Design review of the part built by this model. Coordinates are the model's own, in mm. A direction names the side the tool comes from. Give positions to 0.01 mm unless a question says otherwise; leave off trailing zeros. Order: outer loops, then holes, each group sorted by start corner. A loop starts at its lowest first (then second) coordinate and runs counter-clockwise, first axis right, second up. Notation, with made-up numbers: M 31,15 L 90,15 A37 cw 90,52 Z; hole C 85.5,-25.75 d9. An arc over 180 degrees is marked long. Answer as a JSON object with one key per item and string values.
from build123d import *

# Parameters (mm, degrees)
CREATE_PROFILE_DEPTH     = 38
CUT_SHACKLE_HOLE_DEPTH   = 160.753716702
ROUND_EDGES_R            = 10
UNECESSARY_CHAMFERS_SIZE = 1.5


with BuildPart() as part:
    # Sketch1 → Create profile (new body)
    with BuildSketch(Plane(origin=(0, 0, 0), x_dir=(1, 0, 0), z_dir=(0, 1, 0))):
        with BuildLine():
            Line((0, 0), (0, 56))
            Line((0, 56), (96.5, 56))
            Line((96.5, 56), (118.5, 45))
            Line((118.5, 45), (148.5, 45))
            Line((148.5, 45), (148.5, 37))
            Line((148.5, 37), (118.5, 37))
            Line((118.5, 37), (96.5, 30))
            Line((96.5, 30), (92.5, 30))
            Line((92.5, 30), (92.5, 41.464466094))
            ThreePointArc((92.5, 41.464466094), (92.5, 45), (88.964466094, 45))
            Line((88.964466094, 45), (64.25, 45))
            Line((64.25, 45), (61.25, 48))
            Line((61.25, 48), (51.25, 48))
            Line((51.25, 48), (48.25, 45))
            Line((48.25, 45), (23.535533906, 45))
            ThreePointArc((23.535533906, 45), (20, 45), (20, 41.464466094))
            Line((20, 41.464466094), (20, 0))
            Line((20, 0), (0, 0))
        make_face()
    extrude(amount=CREATE_PROFILE_DEPTH)

    # Sketch3 → Cut shackle hole (cut, through all)
    with BuildSketch(Plane(origin=(0, 0, -45), x_dir=(-1, 0, 0), z_dir=(0, 0, -1))):
        with BuildLine():
            Line((-134, 28), (-134, 10))
            ThreePointArc((-134, 10), (-138, 6), (-142, 10))
            Line((-142, 10), (-142, 28))
            ThreePointArc((-142, 28), (-138, 32), (-134, 28))
        make_face()
    extrude(amount=-CUT_SHACKLE_HOLE_DEPTH, mode=Mode.SUBTRACT)

    # Round Edges
    round_edges_edges = [part.edges().sort_by_distance(p)[0] for p in [
        (148.5, 0, -41),
        (148.5, 38, -41),
    ]]
    fillet(round_edges_edges, radius=ROUND_EDGES_R)

    # Unecessary chamfers
    unecessary_chamfers_edges = [part.edges().sort_by_distance(p)[0] for p in [
        (20, 38, -45),
        (35.892766953, 38, -45),
        (0, 0, -28),
        (48.25, 0, -56),
        (107.5, 0, -50.5),
        (128.5, 0, -37),
        (107.5, 0, -33.5),
        (94.5, 0, -30),
        (92.5, 0, -35.732233047),
        (49.75, 38, -46.5),
        (92.5, 0, -45),
        (76.607233047, 0, -45),
        (62.75, 0, -46.5),
        (56.25, 0, -48),
        (49.75, 0, -46.5),
        (35.892766953, 0, -45),
        (20, 0, -45),
        (20, 0, -20.732233047),
        (10, 0, 0),
        (56.25, 38, -48),
        (62.75, 38, -46.5),
        (0, 19, 0),
        (0, 19, -56),
        (92.5, 19, -30),
        (20, 19, 0),
        (76.607233047, 38, -45),
        (92.5, 38, -45),
        (92.5, 38, -35.732233047),
        (94.5, 38, -30),
        (107.5, 38, -33.5),
        (10, 38, 0),
        (128.5, 38, -37),
        (138, 32, -37),
        (134, 19, -37),
        (138, 6, -37),
        (142, 19, -37),
        (138, 32, -45),
        (142, 19, -45),
        (138, 6, -45),
        (134, 19, -45),
        (107.5, 38, -50.5),
        (48.25, 38, -56),
        (0, 38, -28),
        (148.5, 19, -45),
        (148.5, 19, -37),
        (128.5, 0, -45),
        (128.5, 38, -45),
        (145.571067812, 35.071067812, -45),
        (145.571067812, 2.928932188, -45),
        (145.571067812, 35.071067812, -37),
        (145.571067812, 2.928932188, -37),
        (20, 38, -20.732233047),
    ]]
    chamfer(unecessary_chamfers_edges, length=UNECESSARY_CHAMFERS_SIZE)


solid = part.part
(1) We need section B-B (z = -12.5). Write out the cut boundary in (x, y), plus the area to 4 significant figures.
Checked values:
{"outline": "M 0,1.5 L 1.5,0 L 18.5,0 L 20,1.5 L 20,36.5 L 18.5,38 L 1.5,38 L 0,36.5 Z", "area": "755.5 mm^2"}
(2) To check wall thickness, follow L1, parallel to X at y = 13, z = -41; L2, parallel to X at y = 26, z = -12.5; L3, parallel to Z at x = 41.5, y = 31. State the ranges of each line that lie inside material, in increasing order. Write a range as from..to.
Checked values:
{"L1": "x = 0..20, 92.5..134, 142..148.5", "L2": "x = 0..20", "L3": "z = -56..-45"}
(3) Insertion check: pin 1 (5 mm diameter, centred on x = 128, y = 10.5, fed in from +Z); pin 2 (5 mm diameter, centred on x = 65.5, y = 19, fed in from +Z); pin 3 (3 mm diameter, centred on x = 55.5, y = 18.5, fed in from +Z). Each pin has a flat end and moves straight along its axis. Give the tip position at first contact, or say it passes through.
Checked values:
{"pin 1": "stops at z = -37", "pin 2": "stops at z = -45", "pin 3": "stops at z = -48"}
(4) Draft analysis for pull direction Y (two halves, no side actions). For faces 5 (the flat face through (50, 38, -50)), 6 (the conical face through (19.87, 1.26, -45.21)), 7 (the conical face through (137.9, 5.8, -43.7)), state which applies: +Y half, -Y half, draft (parallel to the pull), parting line (faces both ways), or undercut.
Checked values:
{"face 5": "+Y half", "face 6": "-Y half", "face 7": "undercut"}
(5) Tool access review of faces 1 (the flat face through (56, 19, -48)), 2 (the conical face through (138.1, 32.2, -43.7)), 3 (the flat face through (49.47, 0.76, -47.27)), 4 (the flat face through (49.456, 37.26, -47.282)): name each direction out of +Z, -Z, +X, -X, +Y, -Y from which nothing blocks a thin tool from reaching the whole face with its end or side.
Checked values:
{"face 1": "+Z, +Y, -Y", "face 2": "-Z", "face 3": "+Z, -Y", "face 4": "+Z, +Y"}
(6) We need section C-C (x = 102). Write out the cut boundary in (y, z), plus the area to 3 significant figures.
Checked values:
{"outline": "M 0,-51.57 L 1.5,-53.25 L 36.5,-53.25 L 38,-51.57 L 38,-33.32 L 36.5,-31.75 L 1.5,-31.75 L 0,-33.32 Z", "area": "812 mm^2"}
